from build123d import *

# Parameters (mm, degrees)
F0_W     = 60
F0_H     = 60
F0_R     = 3.862791
F0_R_2   = 1.5
F0_W_2   = 12
F0_H_2   = 11
F1_DEPTH = 4
F2_R     = 2
F3_DEPTH = 25
F4_R     = 5
F5_R     = 1


with BuildPart() as f1:
    # F0 (on Top) → F1 (new body)
    with BuildSketch(Plane.XY):
        Rectangle(F0_W, F0_H)
        with Locations((-18, 0)):
            Circle(F0_R, mode=Mode.SUBTRACT)
        with Locations((-5, 0)):
            Circle(F0_R_2, mode=Mode.SUBTRACT)
        with Locations((10, 0)):
            Rectangle(F0_W_2, F0_H_2, mode=Mode.SUBTRACT)
        with Locations((25, 0)):
            Circle(F0_R_2, mode=Mode.SUBTRACT)
    extrude(amount=F1_DEPTH)

    # F2 (on face) → F3 (cut)
    with BuildSketch(Plane.XY.offset(4)):
        with Locations((-15, 20)):
            Circle(F2_R)
        with Locations((15, 20)):
            Circle(F2_R)
        with Locations((15, -20)):
            Circle(F2_R)
        with Locations((-15, -20)):
            Circle(F2_R)
    extrude(amount=-F3_DEPTH, mode=Mode.SUBTRACT)

    # F4
    f4_edges = [f1.edges().sort_by_distance(p)[0] for p in [
        (-30, 30, 2),
        (-30, -30, 2),
        (30, -30, 2),
        (30, 30, 2),
    ]]
    fillet(f4_edges, radius=F4_R)

    # F5
    f5_edges = [f1.edges().sort_by_distance(p)[0] for p in [
        (4, 5.5, 2),
        (16, 5.5, 2),
        (16, -5.5, 2),
        (4, -5.5, 2),
    ]]
    fillet(f5_edges, radius=F5_R)


solid = f1.part
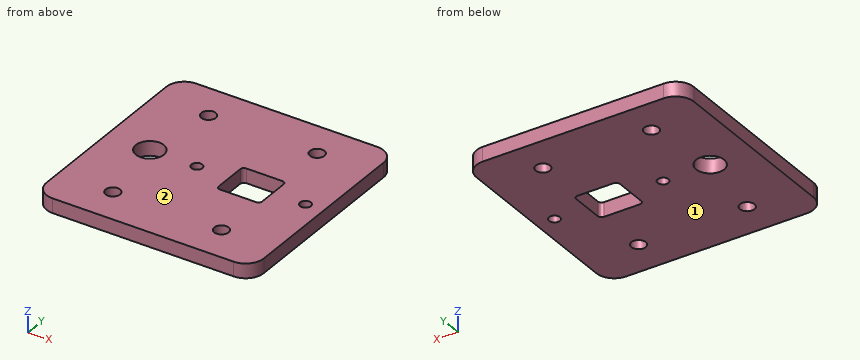
Geometry check sheet. Reference: the model listing, model coordinates, mm. Face numbers are marked on the shaded views. Round coordinates to 2 decimals unless told otherwise and drop trailing zeros. Loops run counter-clockwise (first coordinate to the right, second up) from the corner with the lowest first, then second, coordinate; pieces in that order, holes last.
Item 1: Cross-section at B-B on x = -5. Record the boundary of the cut face in (y, z), then the cut area to 3 significant figures.
Item 2: Mould release check, pull along Z, two halves, no side actions. Record for the marked faces 1 and 2: pulls with the +Z half, pulls with the -Z half, needs draft (parallel to the pull), parting line crosses it, or undercut.
Item 3: Cross-section at C-C on z = 2. Count the separate pieces of the cut face and the enclosed holes in it, then the cut area to 3 significant figures.
Item 4: Thickness scan on line 1 (Y direction, x = 15, z = 1.6); line 2 (Y direction, x = 25, z = 2.25); line 3 (X direction, y = -21, z = 2.2). Record the ranges inside material, lowest first.
Item 5: Cross-section at D-D on y = -20. Record the boundary of the cut face in (x, z).
Item 6: Cross-section at A-A on y = 0. Record the boundary of the cut face in (x, z), then the cut area to 3 significant figures.
Answer sheet:
1. outline: (-30, 0) - (-1.5, 0) - (-1.5, 4) - (-30, 4) - close; (1.5, 0) - (30, 0) - (30, 4) - (1.5, 4) - close
1. area: 228 mm2
2. face 1: pulls with the -Z half
2. face 2: pulls with the +Z half
3. separate pieces: 1
3. enclosed holes: 8
3. area: 3,340 mm2
4. line 1: y = -30 to -22, -18 to -5.5, 5.5 to 18, 22 to 30
4. line 2: y = -30 to -1.5, 1.5 to 30
4. line 3: x = -30 to -16.73, -13.27 to 13.27, 16.73 to 30
5. outline: (-30, 0) - (-17, 0) - (-17, 4) - (-30, 4) - close; (-13, 0) - (13, 0) - (13, 4) - (-13, 4) - close; (17, 0) - (30, 0) - (30, 4) - (17, 4) - close
6. outline: (-30, 0) - (-21.86, 0) - (-21.86, 4) - (-30, 4) - close; (-14.14, 0) - (-6.5, 0) - (-6.5, 4) - (-14.14, 4) - close; (-3.5, 0) - (4, 0) - (4, 4) - (-3.5, 4) - close; (16, 0) - (23.5, 0) - (23.5, 4) - (16, 4) - close; (26.5, 0) - (30, 0) - (30, 4) - (26.5, 4) - close
6. area: 137 mm2
